Drawing for the job (mm, zero at the part's lowest x, y, z). A direction names the side the tool comes from. Coordinates: 2 decimals unless noted, no trailing zeros. Order: outer loops, then holes, each group sorted by start corner. A loop starts at its lowest first (then second) coordinate and runs counter-clockwise, first axis right, second up.
1) Tool access for the marked faces 4 and 5: list every direction of +Z, -Z, +X, -X, +Y, -Y with a clear straight run to the whole face (end or side of a thin tool).
2) Cut at B-B (y = 76). List the corners of the cut face in (x, z).
3) Cut at A-A (x = 42). List the corners of the cut face in (y, z), and give its area (3 significant figures).
4) Wall check: L1, parallel to X at y = 22, z = 29.5; L2, parallel to Y at x = 16.5, z = 2.5; L3, parallel to Z at x = 69.5, y = 74.5. Give the ranges that are in metal, low to high.
5) Cut at C-C (z = 19). List the corners of the cut face in (x, y), and give its area (3 significant figures).
6) Pin check, flat tips, straight feed: pin 1 Ø3 at (x, z) = (123, 6.5) entering from -Y; pin 2 Ø5 at (x, y) = (54, 81.5) entering from -Z. Stop position of each tip, or through.
7) Mould opens along X. For the marked faces 1, 2 and 3 say: +X half, -X half, draft (parallel to the pull), parting line (faces both ways), or undercut.
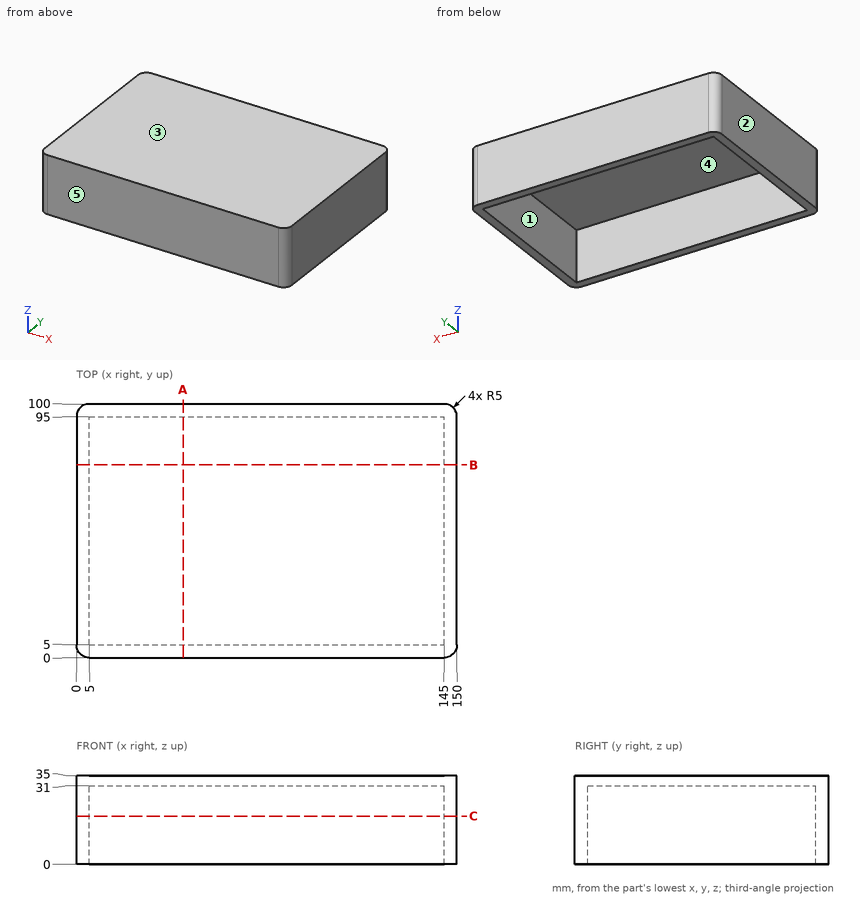
Geometry check:
1. face 4: -Z
1. face 5: +Z, -Z, +X, -X, -Y
2. outline: (0, 0) - (5, 0) - (5, 31) - (145, 31) - (145, 0) - (150, 0) - (150, 35) - (0, 35) - close
3. outline: (0, 0) - (5, 0) - (5, 31) - (95, 31) - (95, 0) - (100, 0) - (100, 35) - (0, 35) - close
3. area: 710 mm2
4. L1: x = 0 to 5, 145 to 150
4. L2: y = 0 to 5, 95 to 100
4. L3: z = 31 to 35
5. outline: (0, 5) arc R5 ccw to (5, 0) - (145, 0) arc R5 ccw to (150, 5) - (150, 95) arc R5 ccw to (145, 100) - (5, 100) arc R5 ccw to (0, 95) - close; hole (5, 5) - (145, 5) - (145, 95) - (5, 95) - close
5. area: 2,380 mm2
6. pin 1: stops at y = 0
6. pin 2: stops at z = 31
7. face 1: undercut
7. face 2: -X half
7. face 3: draft
